Could you check a few things on this model? Use its own coordinates, in mm. A direction names the side the tool comes from. Coordinates: 2 decimals unless noted, no trailing zeros. Loops run counter-clockwise (first coordinate to the right, second up) from the corner with the lowest first, then second, coordinate; pieces in that order, holes last. Notation, with made-up numbers: (-14, -19.75) - (32, -19.75) arc R25 ccw to (32, 5.25) - close; hole circle Ø2 at (64.25, -36). An arc over 180 degrees is marked (long way). Use CSV: the item, a comma, the result in double quotes.
from build123d import *

# Parameters (mm, degrees)
SKETCH1_W           = 50
SKETCH1_H           = 5
BOSS_EXTRUDE1_DEPTH = 70
SKETCH3_R           = 0.95
CUT_EXTRUDE2_DEPTH  = 71


with BuildPart() as part:
    # Sketch1 → Boss-Extrude1 (new body)
    with BuildSketch(Plane.XY):
        with Locations((25, 2.5)):
            Rectangle(SKETCH1_W, SKETCH1_H)
    extrude(amount=BOSS_EXTRUDE1_DEPTH)

    # Sketch3 → Cut-Extrude2 (cut, through all)
    with BuildSketch(Plane.XY.offset(70)):
        with Locations((25, 4.2)):
            Circle(SKETCH3_R)
        Polygon((14, 3.25), (16, 3.25), (16, 1.5), (9, 1.5), (9, 3.25), (11, 3.25), (11, 5), (14, 5), align=None)
        Polygon((41, 3.25), (41, 1.5), (34, 1.5), (34, 3.25), (36, 3.25), (36, 5), (39, 5), (39, 3.25), align=None)
    extrude(amount=-CUT_EXTRUDE2_DEPTH, mode=Mode.SUBTRACT)


solid = part.part
(1) Please list where these lines run through material, in increasing order: line 1 (X direction, y = 4.2, z = 50.5); line 2 (X direction, y = 1.7, z = 5.5); line 3 (Y direction, x = 13.5, z = 56).
Computed:
line 1,"x = 0 to 11, 14 to 24.05, 25.95 to 36, 39 to 50"
line 2,"x = 0 to 9, 16 to 34, 41 to 50"
line 3,"y = 0 to 1.5"
(2) Suppose I cut it at C-C (x = 12). Write out the boundary of the cut face in (y, z).
Computed:
outline,"(0, 0) - (1.5, 0) - (1.5, 70) - (0, 70) - close"
(3) Will this pin go through, and if not, where does the flat tip stop? pin 1 (0.9 mm diameter, centred on y = 4, z = 26, fed in from -X).
Computed:
pin 1,"stops at x = 0"
(4) Suppose I cut it at B-B (z = 41). Write out the boundary of the cut face in (x, y), plus the area to 3 significant figures.
Computed:
outline,"(0, 0) - (50, 0) - (50, 5) - (39, 5) - (39, 3.25) - (41, 3.25) - (41, 1.5) - (34, 1.5) - (34, 3.25) - (36, 3.25) - (36, 5) - (25.51, 5) arc R0.95 cw (long way) to (24.49, 5) - (14, 5) - (14, 3.25) - (16, 3.25) - (16, 1.5) - (9, 1.5) - (9, 3.25) - (11, 3.25) - (11, 5) - (0, 5) - close"
area,"212 mm²"
(5) Thinking about a two-plate mould opening in X: for faces 4 (the face through (35, 3.25, 35)), 5 (the face through (19, 5, 35)), 6 (the face through (0, 2, 35)), which applies, +X half, -X half, draft (parallel to the pull), parting line (faces both ways), or undercut?
Computed:
face 4,"undercut"
face 5,"draft"
face 6,"-X half"
(6) Which directions (+Z, -Z, +X, -X, +Y, -Y) give clear straight access to the entire face, cutting with the end or side of a thin tool? Please do faces 1 (the face through (14, 4, 35)), 2 (the face through (50, 2, 35)), 3 (the face through (34, 2, 35)).
Computed:
face 1,"+Z, -Z, +Y"
face 2,"+Z, -Z, +X, +Y, -Y"
face 3,"+Z, -Z"
(7) Suppose I cut it at A-A (y = 4.2). Write out the boundary of the cut face in (x, z), plus the area to 3 significant figures.
Computed:
outline,"(0, 0) - (11, 0) - (11, 70) - (0, 70) - close; (14, 0) - (24.05, 0) - (24.05, 70) - (14, 70) - close; (25.95, 0) - (36, 0) - (36, 70) - (25.95, 70) - close; (39, 0) - (50, 0) - (50, 70) - (39, 70) - close"
area,"2,950 mm²"
